Geometry check sheet. Reference: the model listing, model coordinates, mm. Face numbers are marked on the shaded views. Give positions to 0.01 mm unless a question says otherwise; leave off trailing zeros. Order: outer loops, then holes, each group sorted by start corner. A loop starts at its lowest first (then second) coordinate and runs counter-clockwise, first axis right, second up. Notation, with made-up numbers: M -2.75,52 L 28.25,52 A12 ccw 28.25,74 Z; hole C -19,18.5 d1. An arc over 180 degrees is marked long. Answer as a JSON object with one key per item and string values. Group by question number.
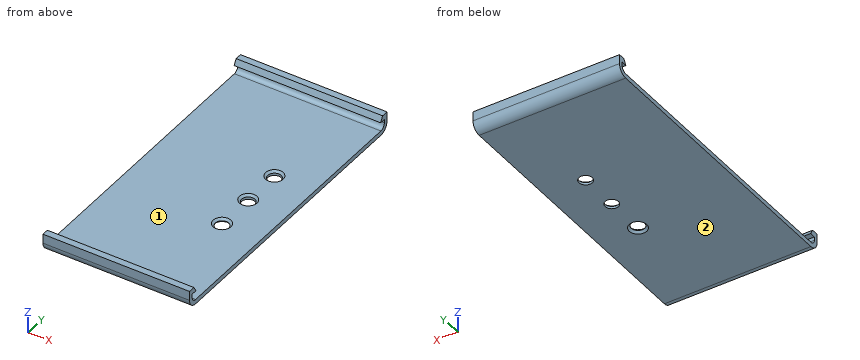
from build123d import *

# Parameters (mm, degrees)
BOSS_EXTRUDE1_DEPTH = 55
CUT_EXTRUDE1_REACH  = 3.7
SKETCH2_R           = 2.5
CHAMFER1_SIZE       = 0.8


with BuildPart() as part:
    # Sketch1 → Boss-Extrude1 (new body)
    with BuildSketch(Plane(origin=(0, 0, 0), x_dir=(0, 0, -1), z_dir=(1, 0, 0))):
        with BuildLine():
            Line((-69.749215448, 110.903184829), (-69.749215448, 113.057885367))
            Line((-69.749215448, 113.057885367), (-68.449215448, 113.057885367))
            ThreePointArc((-68.449215448, 113.057885367), (-67.035001885, 112.47209893), (-66.449215448, 111.057885367))
            Line((-66.449215448, 111.057885367), (-66.449215448, 4.973683681))
            ThreePointArc((-66.449215448, 4.973683681), (-67.035001885, 3.559470118), (-68.449215448, 2.973683681))
            Line((-68.449215448, 2.973683681), (-69.749215448, 2.973683681))
            Line((-69.749215448, 2.973683681), (-69.749215448, 5.128384219))
            Line((-69.749215448, 5.128384219), (-71.749215448, 3.973683681))
            Line((-71.749215448, 3.973683681), (-71.749215448, 1.473683681))
            Line((-71.749215448, 1.473683681), (-68.249215448, 1.473683681))
            ThreePointArc((-68.249215448, 1.473683681), (-65.774341713, 2.498809947), (-64.749215448, 4.973683681))
            Line((-64.749215448, 4.973683681), (-64.749215448, 111.057885367))
            ThreePointArc((-64.749215448, 111.057885367), (-65.774341713, 113.532759101), (-68.249215448, 114.557885367))
            Line((-68.249215448, 114.557885367), (-71.749215448, 114.557885367))
            Line((-71.749215448, 114.557885367), (-71.749215448, 112.057885367))
            Line((-71.749215448, 112.057885367), (-69.749215448, 110.903184829))
        make_face()
    extrude(amount=BOSS_EXTRUDE1_DEPTH)

    # Sketch2 → Cut-Extrude1 (cut, up to next)
    with BuildSketch(Plane.XY.offset(66.449215448), mode=Mode.PRIVATE) as cut_extrude1_sk1:
        with Locations((40, 72.973683681)):
            Circle(SKETCH2_R)
    cut_extrude1_tool1 = extrude(cut_extrude1_sk1.sketch, amount=-CUT_EXTRUDE1_REACH, mode=Mode.PRIVATE) & part.part
    add(cut_extrude1_tool1.solids().sort_by_distance((40, 72.973684, 66.449215))[0], mode=Mode.SUBTRACT)
    # Sketch2 → Cut-Extrude1 (cut, up to next)
    with BuildSketch(Plane.XY.offset(66.449215448), mode=Mode.PRIVATE) as cut_extrude1_sk2:
        with Locations((40, 57.973683681)):
            Circle(SKETCH2_R)
    cut_extrude1_tool2 = extrude(cut_extrude1_sk2.sketch, amount=-CUT_EXTRUDE1_REACH, mode=Mode.PRIVATE) & part.part
    add(cut_extrude1_tool2.solids().sort_by_distance((40, 57.973684, 66.449215))[0], mode=Mode.SUBTRACT)
    # Sketch2 → Cut-Extrude1 (cut, up to next)
    with BuildSketch(Plane.XY.offset(66.449215448), mode=Mode.PRIVATE) as cut_extrude1_sk3:
        with Locations((40, 42.973683681)):
            Circle(SKETCH2_R)
    cut_extrude1_tool3 = extrude(cut_extrude1_sk3.sketch, amount=-CUT_EXTRUDE1_REACH, mode=Mode.PRIVATE) & part.part
    add(cut_extrude1_tool3.solids().sort_by_distance((40, 42.973684, 66.449215))[0], mode=Mode.SUBTRACT)

    # Chamfer1
    chamfer1_edges = [part.edges().sort_by_distance(p)[0] for p in [
        (37.5, 72.973683681, 66.449215448),
        (37.5, 57.973683681, 66.449215448),
        (37.5, 42.973683681, 66.449215448),
        (37.5, 42.973683681, 64.749215448),
    ]]
    chamfer(chamfer1_edges, length=CHAMFER1_SIZE)


solid = part.part
1. Cross-section at C-C (y = 33.5). Record the cut outline in (x, z).
2. Release check for a two-part mould opening along Y. For the marked faces 1 and 2 record: released by +Y, released by -Y, zero draft, split by the parting line, or undercut.
3. Thickness scan on line 1 along Y through (x, z) = (39.5, 68.75); line 2 along Y through (x, z) = (7.5, 68.25); line 3 along Y through (x, z) = (40, 65.6). Record the ranges inside material, lowest first. Write a range as [from, to].
4. Depth check by flat-ended pin: pin 1 (6.5 mm diameter, centred on x = 40, y = 72.97, fed in from -Z); pin 2 (12 mm diameter, centred on x = 43, y = 66.5, fed in from +Z); pin 3 (1.5 mm diameter, centred on y = 60, z = 68.5, fed in from +X). Enter the tip coordinate at first touch or a pass-through.
5. Cross-section at A-A (x = 9). Record the cut outline in (y, z), and give its area (3 significant figures).
6. Cross-section at B-B (x = 40). State how many separate pieces and enclosed holes the cut face has, and give its area (3 significant figures).
Report:
{
 "1": {"outline": "M 0,64.75 L 55,64.75 L 55,66.45 L 0,66.45 Z"},
 "2": {"face 1": "undercut", "face 2": "zero draft"},
 "3": {"line 1": "y = [1.47, 2.97], [113.06, 114.56]", "line 2": "y = [1.47, 2.98], [113.05, 114.56]", "line 3": "y = [2.69, 40.47], [45.47, 55.47], [60.47, 70.47], [75.47, 113.35]"},
 "4": {"pin 1": "stops at z = 64.75", "pin 2": "stops at z = 66.45", "pin 3": "passes through"},
 "5": {"outline": "M 1.47,68.25 A3.5 ccw 4.97,64.75 L 111.06,64.75 A3.5 ccw 114.56,68.25 L 114.56,71.75 L 112.06,71.75 L 110.9,69.75 L 113.06,69.75 L 113.06,68.45 A2 cw 111.06,66.45 L 4.97,66.45 A2 cw 2.97,68.45 L 2.97,69.75 L 5.13,69.75 L 3.97,71.75 L 1.47,71.75 Z", "area": "211 mm2"},
 "6": {"separate pieces": "4", "enclosed holes": "0", "area": "183 mm2"}
}
